Part print with two shaded views. Sizes in mm from the minimum x, y, z corner. A direction names the side the tool comes from. Round coordinates to 2 decimals unless told otherwise and drop trailing zeros. Order: outer loops, then holes, each group sorted by start corner. A loop starts at its lowest first (then second) coordinate and runs counter-clockwise, first axis right, second up. Notation, with made-up numbers: M -3,-17 L 5,-17 A18 ccw 5,18 Z; hole C 57.5,34.25 d11. An arc over 180 degrees is marked long. Return JSON: item names as keys, results as strings. Group by question number.
Item 1: Slice it at D-D on y = 10. Write the cut outline in (x, z), then the cut area to 3 significant figures.
Item 2: Slice it at B-B on x = 12.7. Write the cut outline in (y, z), then the cut area to 3 significant figures.
Item 3: Slice it at C-C on z = 6.25. Write the cut outline in (x, y), then the cut area to 3 significant figures.
Item 4: Slice it at A-A on y = 3. Write the cut outline in (x, z).
Item 5: Probe line 1 along X through (y, z) = (6, 9); line 2 along X through (y, z) = (6.25, 1.5); line 3 along Y through (x, z) = (12.75, 0.5). List the from-to ranges inside material, lowest first.
Item 6: Pin check, flat tips, straight feed: pin 1 Ø1 at (x, y) = (21.5, 11.5) entering from -Z; pin 2 Ø5 at (x, y) = (17, 11.5) entering from -Z; pin 3 Ø3 at (x, z) = (10.5, 7) entering from -Y; pin 4 Ø1.1 at (x, z) = (12.5, 9) entering from -Y. Stop position of each tip, or through.
Item 7: Which spindle directions (+Z, -Z, +X, -X, +Y, -Y) get a long thin tool onto all of the face, cutting with end or side? Do the marked faces 1, 2, 3, 4 and 5. Say none if no direction does.
Item 8: Pull direction X, two halves, no side cores. Call the marked faces 6, 7 and 8: pulls with the +X half, pulls with the -X half, needs draft (parallel to the pull), parting line crosses it, or undercut.
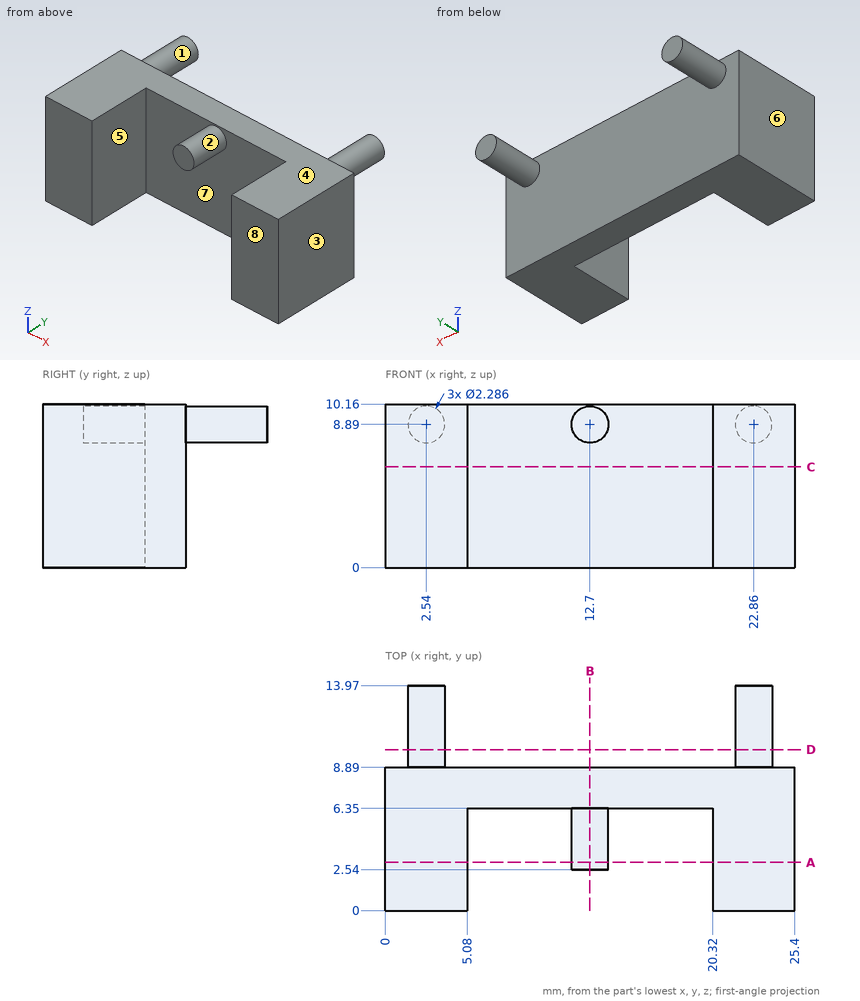
Output values:
{
 "1": {"outline": "C 2.54,8.89 d2.29; C 22.86,8.89 d2.29", "area": "8.21 mm²"},
 "2": {"outline": "M 2.54,7.75 L 6.35,7.75 L 6.35,0 L 8.89,0 L 8.89,10.16 L 6.35,10.16 L 6.35,10.03 L 2.54,10.03 Z", "area": "34.5 mm²"},
 "3": {"outline": "M 0,0 L 5.08,0 L 5.08,6.35 L 20.32,6.35 L 20.32,0 L 25.4,0 L 25.4,8.89 L 0,8.89 Z", "area": "129 mm²"},
 "4": {"outline": "M 0,0 L 5.08,0 L 5.08,10.16 L 0,10.16 Z; C 12.7,8.89 d2.29; M 20.32,0 L 25.4,0 L 25.4,10.16 L 20.32,10.16 Z"},
 "5": {"line 1": "0 to 5.08, 11.56 to 13.84, 20.32 to 25.4", "line 2": "0 to 5.08, 20.32 to 25.4", "line 3": "6.35 to 8.89"},
 "6": {"pin 1": "z = 8.14", "pin 2": "through", "pin 3": "y = 6.35", "pin 4": "y = 2.54"},
 "7": {"face 1": "+Y", "face 2": "-Y", "face 3": "+Z, -Z, +X, +Y, -Y", "face 4": "+Z, +X, -X, +Y, -Y", "face 5": "+Z, -Z, -Y"},
 "8": {"face 6": "pulls with the -X half", "face 7": "undercut", "face 8": "needs draft"}
}
